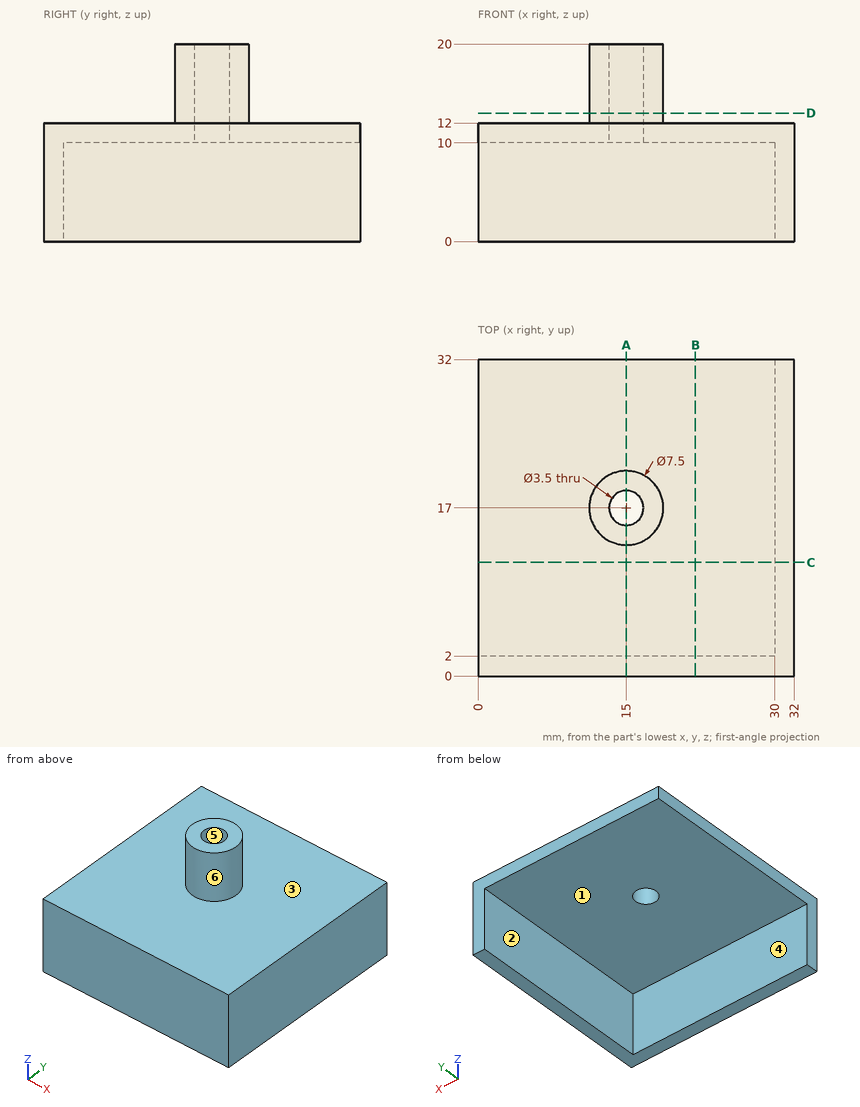
Print and shaded views of the part. All mm, measured from the part's lowest x, y and z. A direction names the side the tool comes from. Coordinates: 2 decimals unless noted, no trailing zeros. Order: outer loops, then holes, each group sorted by start corner. A loop starts at its lowest first (then second) coordinate and runs counter-clockwise, first axis right, second up. Notation, with made-up numbers: (-0.75, 51) - (56.25, 51) arc R24 cw to (56.25, 63) - close; hole circle Ø1 at (63.25, -32.75). An arc over 180 degrees is marked (long way). Return JSON: item names as keys, results as strings. Group by question number.
Item 1: Cut at B-B (x = 22). List the corners of the cut face in (y, z).
Item 2: Cut at D-D (z = 13). List the corners of the cut face in (x, y), plus the area to 3 significant figures.
Item 3: Drill centre lines: probe 1 along Y at (x, z) = (15, 15); probe 2 along Y at (x, z) = (24, 1.75); probe 3 along X at (y, z) = (7, 4.5). Where is each one in solid material? Low to high. Write a range as from..to.
Item 4: Cut at A-A (x = 15). List the corners of the cut face in (y, z), plus the area to 3 significant figures.
Item 5: Pin check, flat tips, straight feed: pin 1 (8 mm diameter, centred on x = 24, y = 9.5, fed in from +Z); pin 2 (3 mm diameter, centred on x = 18, z = 6.5, fed in from +Y); pin 3 (5 mm diameter, centred on x = 13, y = 6.5, fed in from -Z). Stop position of each tip, or through.
Item 6: Pull direction Z, two halves, no side cores. Call the marked faces 1, 2 and 3: pulls with the +Z half, pulls with the -Z half, needs draft (parallel to the pull), parting line crosses it, or undercut.
Item 7: Cut at C-C (y = 11.5). List the corners of the cut face in (x, z), plus the area to 3 significant figures.
Item 8: Which spindle directions (+Z, -Z, +X, -X, +Y, -Y) get a long thin tool onto all of the face, cutting with end or side? Do the marked faces 4, 5 and 6. Say none if no direction does.
Check values:
{
 "1": {"outline": "(0, 0) - (2, 0) - (2, 10) - (32, 10) - (32, 12) - (0, 12) - close"},
 "2": {"outline": "circle Ø7.5 at (15, 17); hole circle Ø3.5 at (15, 17)", "area": "34.6 mm2"},
 "3": {"probe 1": "y = 13.25..15.25, 18.75..20.75", "probe 2": "y = 0..2", "probe 3": "x = 30..32"},
 "4": {"outline": "(0, 0) - (2, 0) - (2, 10) - (15.25, 10) - (15.25, 20) - (13.25, 20) - (13.25, 12) - (0, 12) - close; (18.75, 10) - (32, 10) - (32, 12) - (20.75, 12) - (20.75, 20) - (18.75, 20) - close", "area": "109 mm2"},
 "5": {"pin 1": "stops at z = 12", "pin 2": "stops at y = 2", "pin 3": "stops at z = 10"},
 "6": {"face 1": "pulls with the -Z half", "face 2": "needs draft", "face 3": "pulls with the +Z half"},
 "7": {"outline": "(0, 10) - (30, 10) - (30, 0) - (32, 0) - (32, 12) - (0, 12) - close", "area": "84.0 mm2"},
 "8": {"face 4": "-Z, -X, +Y", "face 5": "+Z, -Z", "face 6": "+Z"}
}
